from build123d import *

# Parameters (mm, degrees)
EXTRUDE_1_DEPTH     = 10
CUT_EXTRUDE_4_DEPTH = 85
SKETCH_6_R          = 1.5
CUT_EXTRUDE_5_DEPTH = 11.953353488
SKETCH_7_R          = 3.25
CUT_EXTRUDE_6_DEPTH = 7.953353488
SKETCH_8_R          = 8
EXTRUDE_2_DEPTH     = 30
SKETCH_9_R          = 3.5
CUT_EXTRUDE_7_DEPTH = 30
SKETCH_10_R         = 5.25
CUT_EXTRUDE_8_DEPTH = 24


with BuildPart() as part:
    # 草图1 → 凸台-拉伸1 (new body)
    with BuildSketch(Plane(origin=(0, 0, 0), x_dir=(1, 0, 0), z_dir=(0, 1, 0))):
        Polygon((-42, 5.5), (-42, 10.5), (42, 10.5), (42, 5.5), (42, -5.5), (31, -5.5), (31, 5.5), (-31, 5.5), (-31, -5.5), (-42, -5.5), align=None)
    extrude(amount=EXTRUDE_1_DEPTH)

    # 草图5 → 切除-拉伸4 (cut, through all)
    with BuildSketch(Plane.ZY.offset(42)):
        Polygon((-5.5, 10), (5.5, 7.052558883), (5.5, 10), align=None)
    extrude(amount=-CUT_EXTRUDE_4_DEPTH, mode=Mode.SUBTRACT)

    # 草图6 → 切除-拉伸5 (cut, through all)
    with BuildSketch(Plane(origin=(0, 12.383949988, -14.397022476), x_dir=(1, 0, 0), z_dir=(0, -0.965925826, -0.258819045))):
        with Locations((-36.5, 14.904894438)):
            Circle(SKETCH_6_R)
        with Locations((36.5, 14.904894438)):
            Circle(SKETCH_6_R)
    extrude(amount=CUT_EXTRUDE_5_DEPTH, mode=Mode.SUBTRACT)

    # 草图7 → 切除-拉伸6 (cut, through all)
    with BuildSketch(Plane(origin=(0, 4.091423714, 1.09629368), x_dir=(1, 0, 0), z_dir=(0, 0.965925826, 0.258819045))):
        with Locations((-36.5, 2.206763503)):
            Circle(SKETCH_7_R)
        with Locations((36.5, 2.206763503)):
            Circle(SKETCH_7_R)
    extrude(amount=-CUT_EXTRUDE_6_DEPTH, mode=Mode.SUBTRACT)

    # 草图8 → 凸台-拉伸2 (add)
    with BuildSketch(Plane.XZ):
        with Locations((0, -13.5)):
            Circle(SKETCH_8_R)
    extrude(amount=-EXTRUDE_2_DEPTH)

    # 草图9 → 切除-拉伸7 (cut)
    with BuildSketch(Plane(origin=(0, 30, 0), x_dir=(1, 0, 0), z_dir=(0, 1, 0))):
        with Locations((0, 13.5)):
            Circle(SKETCH_9_R)
    extrude(amount=-CUT_EXTRUDE_7_DEPTH, mode=Mode.SUBTRACT)

    # 草图10 → 切除-拉伸8 (cut)
    with BuildSketch(Plane.XZ):
        with Locations((0, -13.5)):
            Circle(SKETCH_10_R)
    extrude(amount=-CUT_EXTRUDE_8_DEPTH, mode=Mode.SUBTRACT)


solid = part.part
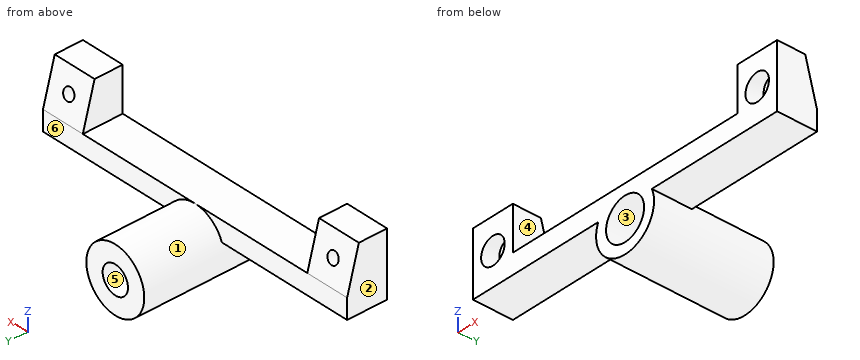
Verification items for the finished model (mm, model axes). Face numbers are marked on the shaded views. A direction names the side the tool comes from. Coordinates: 2 decimals unless noted, no trailing zeros. Order: outer loops, then holes, each group sorted by start corner. A loop starts at its lowest first (then second) coordinate and runs counter-clockwise, first axis right, second up. Notation, with made-up numbers: M 89.5,70.5 L 136.5,70.5 A8 ccw 136.5,76.5 Z; hole C 60,40 d4. An arc over 180 degrees is marked long. One line per item, written item: value. Start each with the question number.
Item 1: Sectioned sample at B-B on y = 12.25. Record the cut outline in (x, z).
Item 2: Depth check by flat-ended pin: P1, Ø5.5, axis at x = -11, z = -7, coming from the +Y side; P2, Ø10, axis at y = 5.5, z = -14.5, coming from the +X side; P3, Ø9.5, axis at x = 0, z = -13.5, coming from the -Y side; P4, Ø3, axis at x = 33, y = 7, coming from the -Z side. Enter the tip coordinate at first touch or a pass-through.
Item 3: Access from +Z, -Z, +X, -X, +Y, -Y to the whole of each face (thin tool, end or side, straight path). Record for the marked faces 4, 5 and 6.
Item 4: Sectioned sample at A-A on z = -13.5. Record the cut outline in (x, y).
Item 5: Sectioned sample at D-D on z = -6.75. Record the cut outline in (x, y), then the cut area to 3 significant figures.
Item 6: Mould release check, pull along X, two halves, no side actions. Record for the marked faces 1, 2 and 3: pulls with the +X half, pulls with the -X half, needs draft (parallel to the pull), parting line crosses it, or undercut.
Item 7: Thickness scan on probe 1 along X at (y, z) = (27.05, -13.5); probe 2 along Z at (x, y) = (0, 14.25); probe 3 along Z at (x, y) = (0, 27.4). Record the ranges inside material, lowest first.
Item 8: Sectioned sample at C-C on x = -13. Record the cut outline in (y, z), then the cut area to 3 significant figures.
Calculated:
1. outline: C 0,-13.5 d16; hole C 0,-13.5 d10.5
2. P1: y = 10
2. P2: x = 42
2. P3: y = 24
2. P4: z = -10.5
3. face 4: +Z, +Y, -Y
3. face 5: +Y, -Y
3. face 6: +Z, +X, +Y
4. outline: M -8,0 L -5.25,0 L -5.25,24 L -3.5,24 L -3.5,30 L -8,30 Z; M 3.5,24 L 5.25,24 L 5.25,0 L 8,0 L 8,30 L 3.5,30 Z
5. outline: M -42,0 L 42,0 L 42,10 L 4.29,10 L 4.29,30 L -4.29,30 L -4.29,10 L -42,10 Z
5. area: 1,010 mm^2
6. face 1: parting line crosses it
6. face 2: pulls with the -X half
6. face 3: undercut
7. probe 1: -8 to -3.5, 3.5 to 8
7. probe 2: -21.5 to -18.75, -8.25 to -5.5
7. probe 3: -21.5 to -17, -10 to -5.5
8. outline: M 0,-10.5 L 10,-10.5 L 10,-5.5 L 0,-5.5 Z
8. area: 50.0 mm^2
